Autodesk Inventor part; units mm, degrees
ref_plane "YZ Plane" through (0, 0, 0) normal (1, 0, 0) x (0, 1, 0)
ref_plane "XZ Plane" through (0, 0, 0) normal (0, 1, 0) x (-1, 0, 0)
ref_plane "XY Plane" through (0, 0, 0) normal (0, 0, 1) x (1, 0, 0)
sketch "Sketch1" plane through (0, 0, 0) normal (0, 1, 0) x (-1, 0, 0)
  circle A0 centre (0, 0) radius 3.429
  line L0 (4.7625, -2.7496) -> (0, -5.4993)
  line L1 (0, -5.4993) -> (-4.7625, -2.7496)
  line L2 (-4.7625, -2.7496) -> (-4.7625, 2.7496)
  line L3 (-4.7625, 2.7496) -> (0, 5.4993)
  line L4 (0, 5.4993) -> (4.7625, 2.7496)
  line L5 (4.7625, 2.7496) -> (4.7625, -2.7496)
  line L6 (4.7625, 0) -> (0, 0) construction
  dimension "d0" = 6.858
  dimension "d1" = 9.525
extrude "Extrusion1" add sketch "Sketch1" along normal blind 1
properties part number "Spacer" material "UHMW, White"
For this review, take the finished solid that the model builds, in its own axes (mm). Round coordinates to 2 decimals unless told otherwise and drop trailing zeros. Loops run counter-clockwise (first coordinate to the right, second up) from the corner with the lowest first, then second, coordinate; pieces in that order, holes last.
Q1. Insertion check: pin 1 Ø1 at (x, z) = (-1, -2) entering from -Y. The pin has a flat end and moves straight along its axis. Give the tip position at first contact, or say it passes through.
Result sheet:
pin 1: passes through
Q2. Add section B-B on x = -0.75. Write out the cut boundary in (y, z).
Result sheet:
outline: (0, -5.07) - (1, -5.07) - (1, -3.35) - (0, -3.35) - close; (0, 3.35) - (1, 3.35) - (1, 5.07) - (0, 5.07) - close
Q3. Add section D-D on x = 4.25. Write out the cut boundary in (y, z), plus the area to 3 significant figures.
Result sheet:
outline: (0, -3.05) - (1, -3.05) - (1, 3.05) - (0, 3.05) - close
area: 6.09 mm2
Q4. To check wall thickness, follow line 1 along Z through (x, y) = (1.25, 0.65); line 2 along X through (y, z) = (0.35, -2.5); line 3 along Z through (x, y) = (-1, 0.55). State the ranges of each line that lie inside material, in increasing order.
Result sheet:
line 1: z = -4.78 to -3.19, 3.19 to 4.78
line 2: x = -4.76 to -2.35, 2.35 to 4.76
line 3: z = -4.92 to -3.28, 3.28 to 4.92
Q5. Mouldability with a two-part tool opening along X and no side actions: class faces 1 (the face through (4.762, 0.5, 0)), 2 (the face through (0.74, 0.49, 3.35)), 3 (the face through (0, 0, -4)) as +X half, -X half, draft (parallel to the pull), parting line (faces both ways), or undercut.
Result sheet:
face 1: +X half
face 2: undercut
face 3: draft
Q6. Add section C-C on y = 0.8. Write out the cut boundary in (x, z), plus the area to 3 significant figures.
Result sheet:
outline: (-4.76, -2.75) - (0, -5.5) - (4.76, -2.75) - (4.76, 2.75) - (0, 5.5) - (-4.76, 2.75) - close; hole circle Ø6.86 at (0, 0)
area: 41.6 mm2
Q7. Add section A-A on z = 0. Write out the cut boundary in (x, y), plus the area to 3 significant figures.
Result sheet:
outline: (-4.76, 0) - (-3.43, 0) - (-3.43, 1) - (-4.76, 1) - close; (3.43, 0) - (4.76, 0) - (4.76, 1) - (3.43, 1) - close
area: 2.67 mm2
